The model under review builds one solid part; all positions refer to its coordinate system, in mm. Face numbers are marked on the shaded views. A direction names the side the tool comes from. Round coordinates to 2 decimals unless told otherwise and drop trailing zeros. Write each loop counter-clockwise with the first axis right and the second up, starting at its lowest first coordinate (ties: lowest second). Pieces come first, ordered by that corner, then holes. Notation, with made-up numbers: (35, -38.5) - (53, -38.5) arc R18 ccw to (53, -30.5) - close; hole circle Ø1 at (24.5, 13.25). An arc over 180 degrees is marked (long way). Use one line per item in the form item = value.
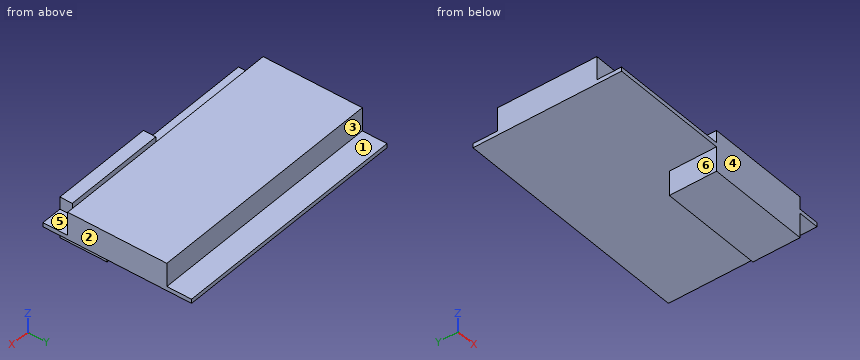
from build123d import *

# Parameters (mm, degrees)
SKETCH_1_W      = 98.25
SKETCH_1_H      = 60.1
EXTRUDE_1_DEPTH = 1.7
SKETCH_2_W      = 98.25
SKETCH_2_H      = 40.1
EXTRUDE_2_DEPTH = 9.5
SKETCH_3_W      = 42
SKETCH_3_H      = 5
EXTRUDE_3_DEPTH = 5
SKETCH_4_W      = 42
SKETCH_4_H      = 19.1
EXTRUDE_4_DEPTH = 10


with BuildPart() as part:
    # Эскиз1 → Бобышка-Вытянуть1 (new body)
    with BuildSketch(Plane.XY):
        with Locations((49.125, 30.05)):
            Rectangle(SKETCH_1_W, SKETCH_1_H)
    extrude(amount=EXTRUDE_1_DEPTH)

    # Эскиз2 → Бобышка-Вытянуть2 (add)
    with BuildSketch(Plane.XY.offset(1.7)):
        with Locations((49.125, 30.05)):
            Rectangle(SKETCH_2_W, SKETCH_2_H)
    extrude(amount=EXTRUDE_2_DEPTH)

    # Эскиз3 → Бобышка-Вытянуть3 (add)
    with BuildSketch(Plane.XY.offset(1.7)):
        with Locations((68.75, 2.5)):
            Rectangle(SKETCH_3_W, SKETCH_3_H)
    extrude(amount=EXTRUDE_3_DEPTH)

    # Эскиз4 → Бобышка-Вытянуть4 (add)
    with BuildSketch(Plane(origin=(0, 0, 0), x_dir=(-1, 0, 0), z_dir=(0, 0, -1))):
        with Locations((-68.75, 9.55)):
            Rectangle(SKETCH_4_W, SKETCH_4_H)
    extrude(amount=EXTRUDE_4_DEPTH)


solid = part.part
(1) Add section A-A on y = 14.5. Write out the cut boundary in (x, z).
Geometry results:
outline = (0, 0) - (47.75, 0) - (47.75, -10) - (89.75, -10) - (89.75, 0) - (98.25, 0) - (98.25, 11.2) - (0, 11.2) - close
(2) Machinability: for the marked faces 1 and 2, which of the approach directions +Z, -Z, +X, -X, +Y, -Y give a long, thin tool a straight path to every point of the face, cutting with its end or side? Answer none if there is none.
Geometry results:
face_1 = +Z, +X, -X, +Y
face_2 = +Z, -Z, +X, +Y, -Y
(3) Add section B-B on x = 77.5. Write out the cut boundary in (y, z).
Geometry results:
outline = (0, -10) - (19.1, -10) - (19.1, 0) - (60.1, 0) - (60.1, 1.7) - (50.1, 1.7) - (50.1, 11.2) - (10, 11.2) - (10, 1.7) - (5, 1.7) - (5, 6.7) - (0, 6.7) - close
(4) The part is to be moulded in two halves that separate along Y. For the marked faces 3, 4, 5 and 6, say which applies: +Y half, -Y half, draft (parallel to the pull), parting line (faces both ways), or undercut.
Geometry results:
face_3 = +Y half
face_4 = -Y half
face_5 = undercut
face_6 = draft
(5) To check wall thickness, follow L1, parallel to Y at x = 89, z = 6; L2, parallel to Y at x = 35.5, z = 7; L3, parallel to Z at x = 88.5, y = 42.5. State the ranges of each line that lie inside material, in increasing order.
Geometry results:
L1 = 0 to 5, 10 to 50.1
L2 = 10 to 50.1
L3 = 0 to 11.2
(6) Add section C-C on z = -8. Write out the cut boundary in (x, y), then the cut area to 3 significant figures.
Geometry results:
outline = (47.75, 0) - (89.75, 0) - (89.75, 19.1) - (47.75, 19.1) - close
area = 802 mm2
(7) Insertion check: P1, Ø2.5, axis at x = 65.5, y = 2.5, coming from the +Z side; P2, Ø2.5, axis at y = 3.5, z = 5, coming from the +X side; P3, Ø8, axis at y = 14, z = -4.5, coming from the -X side. Each pin has a flat end and moves straight along its axis. Give the tip position at first contact, or say it passes through.
Geometry results:
P1 = 6.7
P2 = 89.75
P3 = 47.75
(8) Add section D-D on y = 4. Write out the cut boundary in (x, z).
Geometry results:
outline = (0, 0) - (47.75, 0) - (47.75, -10) - (89.75, -10) - (89.75, 0) - (98.25, 0) - (98.25, 1.7) - (89.75, 1.7) - (89.75, 6.7) - (47.75, 6.7) - (47.75, 1.7) - (0, 1.7) - close
